The figure shows three views and two pictorial views of one solid part (mm, origin at its lowest corner). Answer the questions. Give positions to 0.01 mm unless a question says otherwise; leave off trailing zeros. Loops run counter-clockwise (first coordinate to the right, second up) from the corner with the lowest first, then second, coordinate; pieces in that order, holes last. Notation, with made-up numbers: (19, 1.25) - (71, 1.25) arc R21 cw to (71, 35.25) - close; hole circle Ø7 at (-15, 86). An arc over 180 degrees is marked (long way). Write each question's results on one line, items separated by ' | '.
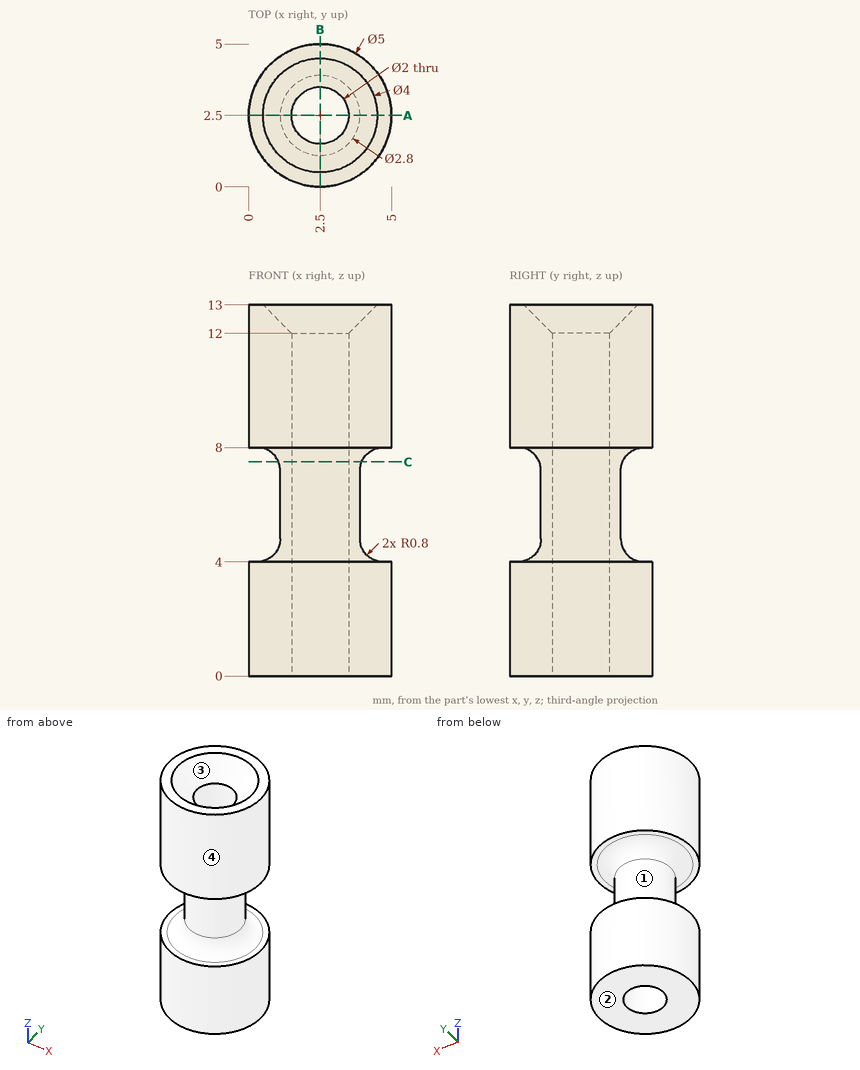
Item 1: Find the intervals of material crossed by line 1 along Y through (x, z) = (2.5, 6.75); line 2 along Y through (x, z) = (2.5, 3.5); line 3 along Z through (x, y) = (0.6, 3.9), in increasing order. Write a range as [from, to].
Values found:
line 1: y = [1.1, 1.5], [3.5, 3.9] | line 2: y = [0, 1.5], [3.5, 5] | line 3: z = [0, 4], [8, 13]
Item 2: A flat-ended cylindrical pin translates along its axis: P1, Ø1.5, axis at x = 2.5, y = 3, coming from the +Z side. Find the tip coordinate at first contact, or state that the pin passes through.
Values found:
P1: stops at z = 12.25
Item 3: For a pull along Z with two mould halves and no side action, classify the marked faces 1, 2, 3 and 4 as released by +Z, released by -Z, zero draft, split by the parting line, or undercut.
Values found:
face 1: undercut | face 2: released by -Z | face 3: released by +Z | face 4: zero draft
Item 4: A cutting plane is placed at A-A, the plane y = 2.5. Determine the outline of the cut face in (x, z), plus the area to 3 significant figures.
Values found:
outline: (0, 0) - (1.5, 0) - (1.5, 12) - (0.5, 13) - (0, 13) - (0, 8) - (0.3, 8) arc R0.8 cw to (1.1, 7.2) - (1.1, 4.8) arc R0.8 cw to (0.3, 4) - (0, 4) - close; (3.5, 0) - (5, 0) - (5, 4) - (4.7, 4) arc R0.8 cw to (3.9, 4.8) - (3.9, 7.2) arc R0.8 cw to (4.7, 8) - (5, 8) - (5, 13) - (4.5, 13) - (3.5, 12) - close | area: 29.7 mm²
Item 5: A cutting plane is placed at C-C, the plane z = 7.5. Determine the outline of the cut face in (x, y), plus the area to 3 significant figures.
Values found:
outline: circle Ø2.92 at (2.5, 2.5); hole circle Ø2 at (2.5, 2.5) | area: 3.54 mm²
